For this review, take the finished solid that the model builds, in its own axes (mm). Face numbers are marked on the shaded views. A direction names the side the tool comes from. Round coordinates to 2 decimals unless told otherwise and drop trailing zeros. Loops run counter-clockwise (first coordinate to the right, second up) from the corner with the lowest first, then second, coordinate; pieces in that order, holes last. Notation, with made-up numbers: (51, 7.25) -> (60, 7.25) arc R13 ccw to (60, 19.25) -> close; hole circle Ø6 at (38.25, -33.75). An arc over 180 degrees is marked (long way). Use one line per item in the form item = value. Start each with the question number.
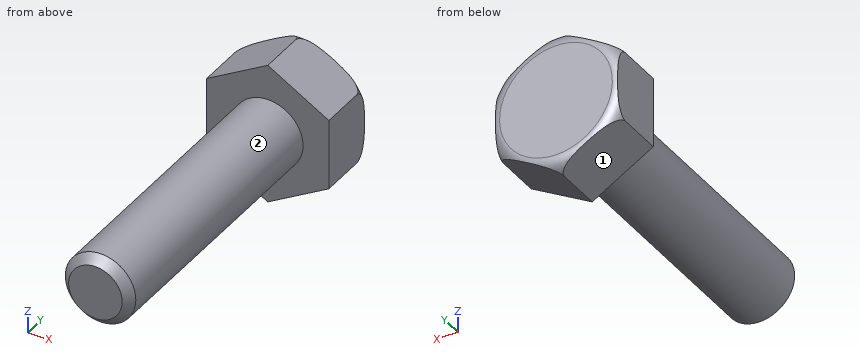
from build123d import *

# Parameters (mm, degrees)
EXTRUDE1_DEPTH = 5.334
SKETCH3_R      = 3.175
EXTRUDE2_DEPTH = 25.4
CHAMFER1_SIZE  = 0.762


with BuildPart() as part:
    # Sketch1 → Extrude1 (new body)
    with BuildSketch(Plane(origin=(0, 0, 0), x_dir=(1, 0, 0), z_dir=(0, 1, 0))):
        Polygon((0, 6.35), (-5.499261314, 3.175), (-5.499261314, -3.175), (0, -6.35), (5.499261314, -3.175), (5.499261314, 3.175), align=None)
    extrude(amount=EXTRUDE1_DEPTH)

    # Sketch3 → Extrude2 (add)
    with BuildSketch(Plane.XZ):
        Circle(SKETCH3_R)
    extrude(amount=EXTRUDE2_DEPTH)

    # Sketch2 → Cut-Revolve1 (revolve, cut)
    with BuildSketch(Plane(origin=(0, 0, 0), x_dir=(0, 0, -1), z_dir=(1, 0, 0))):
        with BuildLine():
            Line((5.08, 5.334), (6.35, 5.334))
            Line((6.35, 5.334), (6.35, 4.064))
            ThreePointArc((6.35, 4.064), (5.978025612, 4.962025612), (5.08, 5.334))
        make_face()
    revolve(axis=Axis((0, -25.4, 0), (0, 1, 0)), mode=Mode.SUBTRACT)

    # Chamfer1
    chamfer1_edges = [part.edges().sort_by_distance(p)[0] for p in [
        (-3.175, -25.4, 0),
    ]]
    chamfer(chamfer1_edges, length=CHAMFER1_SIZE)


solid = part.part
Item 1: Take a section at A-A on y = -19. Give the boundary of the cut face in (x, z) (3 decimals), plus the area to 3 significant figures.
Item 2: Wall thickness on line 1 (Y direction, x = 1, z = -3.5); line 2 (Z direction, x = 1, y = -3); line 3 (Y direction, x = 4.5, z = -3.5): over which ranges is each line inside the solid? List them lowest first.
Item 3: Machinability: for the marked faces 1 and 2, which of the approach directions +Z, -Z, +X, -X, +Y, -Y give a long, thin tool a straight path to every point of the face, cutting with its end or side? Answer none if there is none.
Item 4: For P1, Ø1.5, axis at y = -8, z = 0, coming from the -X side (3 decimals); P2, Ø2, axis at x = -3, z = -2.5, coming from the -Y side; P3, Ø1.5, axis at y = -2, z = 2, coming from the +X side, all flat-tipped, find the tip position at first contact; note any pin that passes through.
Results:
q1.outline = circle Ø6.35 at (0, 0)
q1.area = 31.7 mm2
q2.line_1 = 0 to 5.33
q2.line_2 = -3.01 to 3.01
q2.line_3 = 0 to 5.17
q3.face_1 = -Z, -X, +Y, -Y
q3.face_2 = -Y
q4.P1 = -3.175
q4.P2 = -24.91
q4.P3 = 2.92
